Read the model definition and answer for the solid it produces. Units are mm, in the model's axes. Coordinates: 2 decimals unless noted, no trailing zeros. Write each loop counter-clockwise with the first axis right and the second up, starting at its lowest first coordinate (ties: lowest second). Pieces come first, ordered by that corner, then holes. Notation, with made-up numbers: (54.5, -28.75) -> (98.5, -28.75) arc R10 ccw to (98.5, -10.75) -> close; hole circle Ø6 at (-20, 25). An arc over 180 degrees is marked (long way). One line per item, written item: value. Start each with the question number.
1. Find section A-A, the plane z = -39.5. Write down the section's boundary in (x, y).
2. Find section B-B, the plane y = 0.9. State how many separate pieces and enclosed holes the cut face has, and give its area (3 significant figures).
3. Consider line 1 along X through (y, z) = (1.9, -9.5); line 2 along X through (y, z) = (1.35, -74); line 3 along Z through (x, y) = (41, 1.2). Determine where each line is inside the solid, lowest interval first.
4. Find section C-C, the plane x = 42. Write down the section's boundary in (y, z).
5. Given P1, Ø4.5, axis at x = 72.517, z = -72.517, coming from the +Y side, flat-ended and moving along its own axis, determine where the tip first touches the part or whether it passes through.
```python
from build123d import *

# Parameters (mm, degrees)
SKETCH1_W           = 82.042
SKETCH1_H           = 82.042
BOSS_EXTRUDE1_DEPTH = 2
SKETCH2_R           = 2
CUT_EXTRUDE1_DEPTH  = 3
SKETCH3_R           = 12.5476
CUT_EXTRUDE2_DEPTH  = 3


with BuildPart() as part:
    # Sketch1 → Boss-Extrude1 (new body)
    with BuildSketch(Plane(origin=(0, 0, 0), x_dir=(1, 0, 0), z_dir=(0, 1, 0))):
        with Locations((41.021, 41.021)):
            Rectangle(SKETCH1_W, SKETCH1_H)
    extrude(amount=BOSS_EXTRUDE1_DEPTH)

    # Sketch2 → Cut-Extrude1 (cut, through all)
    with BuildSketch(Plane(origin=(0, 2, 0), x_dir=(-1, 0, 0), z_dir=(0, 1, 0))):
        with Locations((-28.321, -53.721)):
            Circle(SKETCH2_R)
        with Locations((-53.721, -53.721)):
            Circle(SKETCH2_R)
        with Locations((-53.721, -28.321)):
            Circle(SKETCH2_R)
        with Locations((-28.321, -28.321)):
            Circle(SKETCH2_R)
        with Locations((-9.525, -9.525)):
            Circle(SKETCH2_R)
        with Locations((-9.525, -72.517)):
            Circle(SKETCH2_R)
        with Locations((-72.517, -9.525)):
            Circle(SKETCH2_R)
        with Locations((-72.517, -72.517)):
            Circle(SKETCH2_R)
    extrude(amount=-CUT_EXTRUDE1_DEPTH, mode=Mode.SUBTRACT)

    # Sketch3 → Cut-Extrude2 (cut, through all)
    with BuildSketch(Plane(origin=(0, 2, 0), x_dir=(1, 0, 0), z_dir=(0, 1, 0))):
        with Locations((41.021, 41.021)):
            Circle(SKETCH3_R)
    extrude(amount=-CUT_EXTRUDE2_DEPTH, mode=Mode.SUBTRACT)


solid = part.part
```
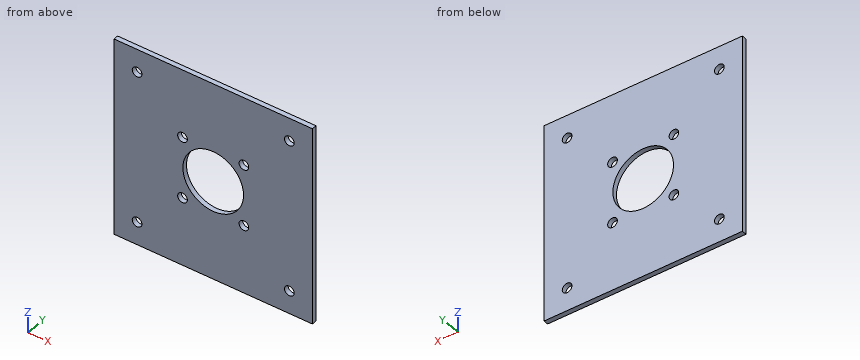
Answer block:
1. outline: (0, 0) -> (28.57, 0) -> (28.57, 2) -> (0, 2) -> close; (53.48, 0) -> (82.04, 0) -> (82.04, 2) -> (53.48, 2) -> close
2. separate pieces: 1
2. enclosed holes: 9
2. area: 6,140 mm2
3. line 1: x = 0 to 7.53, 11.52 to 70.52, 74.52 to 82.04
3. line 2: x = 0 to 8.18, 10.87 to 71.18, 73.86 to 82.04
3. line 3: z = -82.04 to -53.57, -28.47 to 0
4. outline: (0, -82.04) -> (2, -82.04) -> (2, -53.53) -> (0, -53.53) -> close; (0, -28.51) -> (2, -28.51) -> (2, 0) -> (0, 0) -> close
5. P1: stops at y = 2
